from build123d import *

# Parameters (mm, degrees)
F0_R     = 14
F0_R_2   = 1.75
F0_R_3   = 5.1
F1_DEPTH = 10
F6_DEPTH = 40


with BuildPart() as f1:
    # F0 (on Top) → F1 (new body)
    with BuildSketch(Plane.XY):
        Circle(F0_R)
        with Locations((0, -8)):
            Circle(F0_R_2, mode=Mode.SUBTRACT)
        with Locations((-9.5, 0)):
            Circle(F0_R_2, mode=Mode.SUBTRACT)
        Circle(F0_R_3, mode=Mode.SUBTRACT)
        with Locations((9.5, 0)):
            Circle(F0_R_2, mode=Mode.SUBTRACT)
        with Locations((0, 8)):
            Circle(F0_R_2, mode=Mode.SUBTRACT)
    extrude(amount=F1_DEPTH)

    # F5 (on face) → F6 (intersect)
    with BuildSketch(Plane(origin=(17.6564226245, -17.6564226245, -1.2253490154), x_dir=(0.7045622489, 0.7079556371, -0.0488963521), z_dir=(0.706256905, -0.706256905, -0.0490139606))):
        Polygon((-42.6054166353, 4.1487906781), (-42.3605061004, -0.8479598781), (14.9219552549, 1.9596804268), (14.7750896798, 4.9560833541), align=None)
        Polygon((14.7750896798, 4.9560833541), (14.9219552549, 1.9596804268), (100.7277084193, 6.1653602332), align=None)
    extrude(amount=-F6_DEPTH, mode=Mode.INTERSECT)


solid = f1.part
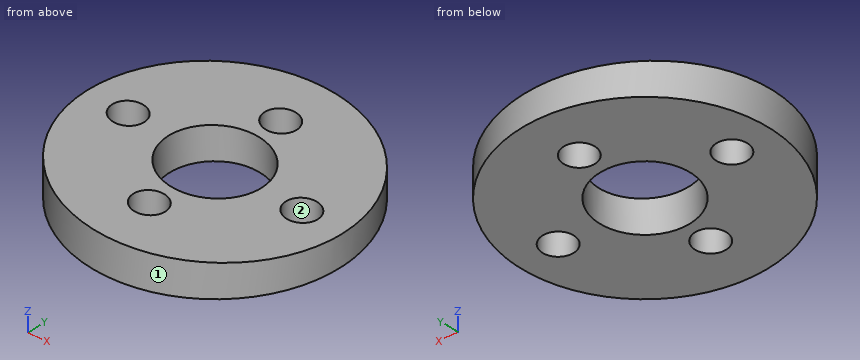
Check sheet for the modelled part. Datum: model origin and axes. Units: mm. Face numbers are marked on the shaded views. Coordinates: 2 decimals unless noted, no trailing zeros. Write each loop counter-clockwise with the first axis right and the second up, starting at its lowest first coordinate (ties: lowest second). Pieces come first, ordered by that corner, then holes. Notation, with made-up numbers: M 76,60 L 111,60 A21 cw 111,90 Z; hole C 59.5,34.5 d1. An arc over 180 degrees is marked long. Answer as CSV lines item,"result".
Q1. Material ranges on probe 1 along Y at (x, z) = (0, 1.8); probe 2 along X at (y, z) = (0, 3.45); probe 3 along X at (y, z) = (1.5, 2.65), recorded low to high. Write a range as from..to.
Check result:
probe 1,"-14..-9.75, -6.25..-5.1, 5.1..6.25, 9.75..14"
probe 2,"-14..-11.25, -7.75..-5.1, 5.1..7.75, 11.25..14"
probe 3,"-13.92..-10.4, -8.6..-4.87, 4.87..8.6, 10.4..13.92"
Q2. Cross-section at C-C (z = 2.25). Record the boundary of the cut face in (x, y), then the cut area to 3 significant figures.
Check result:
outline,"C 0,0 d28; hole C -9.5,0 d3.5; hole C 0,0 d10.2; hole C 0,-8 d3.5; hole C 0,8 d3.5; hole C 9.5,0 d3.5"
area,"496 mm^2"
Q3. Go/stop test with flat-tipped pins: pin 1 (3 mm diameter, centred on x = -3, y = 10.5, fed in from +Z); pin 2 (12 mm diameter, centred on x = -8, y = 11, fed in from +Z); pin 3 (5 mm diameter, centred on x = 6, y = 10, fed in from +Z). Record where each tip stops, or that it passes through.
Check result:
pin 1,"z = 5.13"
pin 2,"z = 5.55"
pin 3,"z = 4.65"
Q4. Cross-section at B-B (y = 1.25). Record the boundary of the cut face in (x, z).
Check result:
outline,"M -13.94,1.76 L -10.72,1.64 L -10.72,5.41 L -13.94,5.6 Z; M -8.28,1.56 L -4.94,1.44 L -4.94,5.06 L -8.28,5.26 Z; M 4.94,1.1 L 8.28,0.98 L 8.28,4.28 L 4.94,4.48 Z; M 10.72,0.9 L 13.94,0.79 L 13.94,3.94 L 10.72,4.13 Z"
Q5. Cross-section at D-D (x = 1.25). Record the boundary of the cut face in (y, z), then the cut area to 3 significant figures.
Check result:
outline,"M -13.94,0.7 L -9.22,0.86 L -9.22,4.59 L -13.94,4.54 Z; M -6.78,0.95 L -4.94,1.01 L -4.94,4.63 L -6.78,4.61 Z; M 4.94,1.36 L 6.78,1.42 L 6.78,4.75 L 4.94,4.73 Z; M 9.22,1.51 L 13.94,1.67 L 13.94,4.82 L 9.22,4.77 Z"
area,"45.8 mm^2"
Q6. Mould release check, pull along X, two halves, no side actions. Record for the marked faces 1 and 2: released by +X, released by -X, zero draft, split by the parting line, or undercut.
Check result:
face 1,"split by the parting line"
face 2,"undercut"
Q7. Cross-section at A-A (x = 9.5). Record the boundary of the cut face in (y, z), then the cut area to 3 significant figures.
Check result:
outline,"M -10.28,0.54 L -1.75,0.84 L -1.75,4.17 L -10.28,4.09 Z; M 1.75,0.96 L 10.28,1.26 L 10.28,4.29 L 1.75,4.21 Z"
area,"56.2 mm^2"
